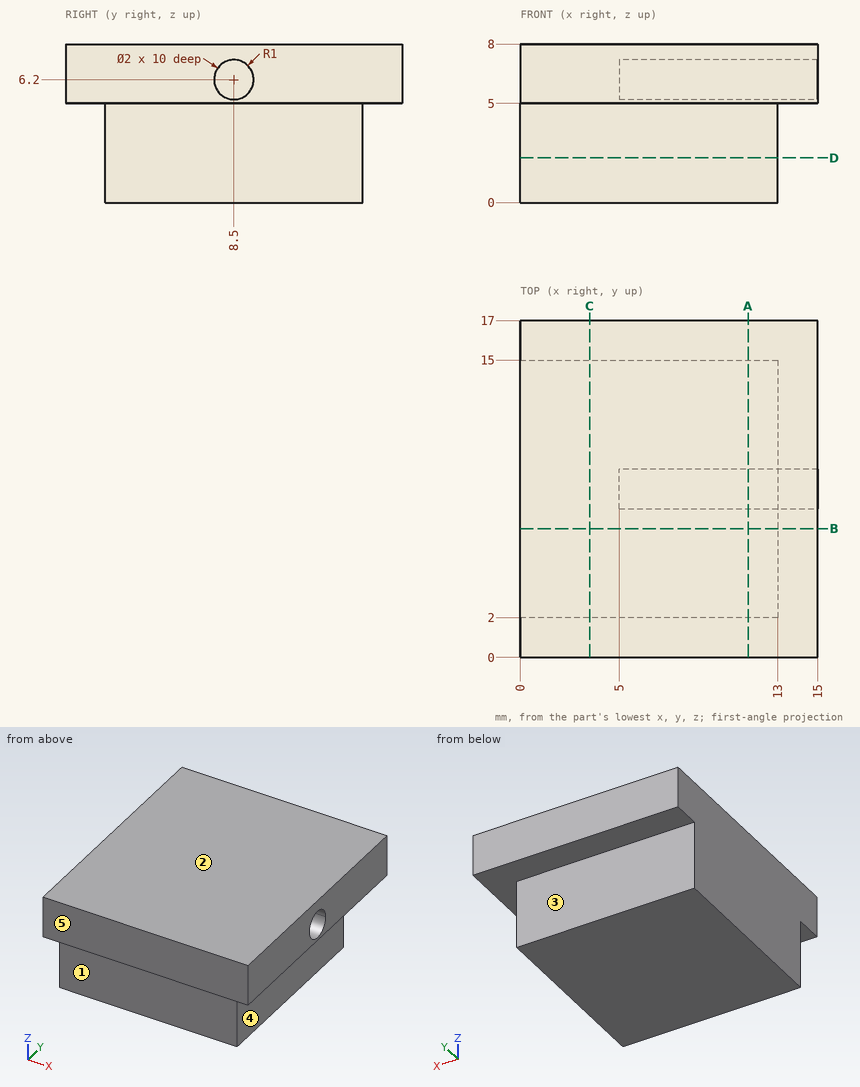
Can you work these out from the drawing? Everything is in mm from the part's minimum corner. A direction names the side the tool comes from. Round coordinates to 2 decimals unless told otherwise and drop trailing zeros. Write each loop counter-clockwise with the first axis right and the second up, starting at its lowest first coordinate (ties: lowest second). Pieces come first, ordered by that corner, then holes.
1. For the marked faces 1, 2, 3, 4 and 5, which set-ups out of +Z, -Z, +X, -X, +Y, -Y let a thin tool reach every point of the face, with its end or its side?
2. Suppose I cut it at A-A (x = 11.5). List the corners of the cut face in (y, z) for me, and give its area (3 significant figures).
3. Suppose I cut it at B-B (y = 6.5). List the corners of the cut face in (x, z) for me, and give its area (3 significant figures).
4. Suppose I cut it at D-D (z = 2.25). List the corners of the cut face in (x, y) for me, and give its area (3 significant figures).
5. I need wall thicknesses on L1, parallel to Z at x = 7.75, y = 8.5; L2, parallel to Y at x = 9.25, z = 6.2; L3, parallel to Y at x = 3.25, z = 2.5. Which ranges of each line are inside material? Lowest first, please.
6. Suppose I cut it at C-C (x = 3.5). List the corners of the cut face in (y, z) for me.
7. Will these pins go through, and if not, where does the flat tip stop? pin 1 Ø2 at (x, y) = (7, 3) entering from -Z; pin 2 Ø1 at (y, z) = (8.5, 6.5) entering from +X; pin 3 Ø2.5 at (x, z) = (4.5, 2) entering from -Y.
Answer sheet:
1. face 1: -Z, +X, -X, -Y
1. face 2: +Z, +X, -X, +Y, -Y
1. face 3: -Z, +X, -X, +Y
1. face 4: -Z, +X, +Y, -Y
1. face 5: +Z, -Z, +X, -X, -Y
2. outline: (0, 5) - (2, 5) - (2, 0) - (15, 0) - (15, 5) - (17, 5) - (17, 8) - (0, 8) - close; hole circle Ø2 at (8.5, 6.2)
2. area: 113 mm2
3. outline: (0, 0) - (13, 0) - (13, 5) - (15, 5) - (15, 8) - (0, 8) - close
3. area: 110 mm2
4. outline: (0, 2) - (13, 2) - (13, 15) - (0, 15) - close
4. area: 169 mm2
5. L1: z = 0 to 5.2, 7.2 to 8
5. L2: y = 0 to 7.5, 9.5 to 17
5. L3: y = 2 to 15
6. outline: (0, 5) - (2, 5) - (2, 0) - (15, 0) - (15, 5) - (17, 5) - (17, 8) - (0, 8) - close
7. pin 1: stops at z = 0
7. pin 2: stops at x = 5
7. pin 3: stops at y = 2
